Here's how the part is built. I have some questions about the finished solid (model axes, mm). A direction names the side the tool comes from. Give positions to 0.01 mm unless a question says otherwise; leave off trailing zeros. Loops run counter-clockwise (first coordinate to the right, second up) from the corner with the lowest first, then second, coordinate; pieces in that order, holes last.
Q1. I'm going to push flat-ended pins straight in: P1, Ø6.5, axis at y = -30, z = -30, coming from the +X side; P2, Ø11, axis at x = 51.5, z = -20.5, coming from the -Y side; P3, Ø4, axis at x = 51, y = -4.5, coming from the -Z side. Where does each tip first touch, or does it pass through?
Q2. For faces 1 (the face through (6, 35, 28.734)), 2 (the face through (16, 17.462, -24)), 3 (the face through (41.275, -8, 13)), which set-ups out of +Z, -Z, +X, -X, +Y, -Y let a thin tool reach every point of the face, with its end or its side?
Q3. I need wall thicknesses on probe 1 along Z at (x, y) = (37.5, -4.5) (1 decimal); probe 2 along Y at (x, z) = (19.5, -31.75); probe 3 along Z at (x, y) = (5.5, 26.5). Which ranges of each line are inside material? Lowest first, please.
Q4. Suppose I cut it at B-B (y = 2). List the corners of the cut face in (x, z) for me (1 decimal), and give its area (3 significant figures).
Q5. Suppose I cut it at A-A (z = 31.75). List the corners of the cut face in (x, y) for me (1 decimal), and give its area (3 significant figures).
Q6. Suppose I cut it at C-C (x = 52). Count the separate pieces of the cut face and the enclosed holes in it, and give its area (3 significant figures).
Q7. Thinking about a two-plate mould opening in Z: for faces 4 (the face through (41.275, -8, -12)), 5 (the face through (48.162, 22.907, 3.495)), 6 (the face through (36, 20.002, -25)), 7 (the face through (6, 28, 20.479)), which applies, pulls with the +Z half, pulls with the -Z half, needs draft (parallel to the pull), parting line crosses it, or undercut?
Autodesk Inventor part; units mm, degrees
ref_plane "YZ Plane" through (0, 0, 0) normal (1, 0, 0) x (0, 1, 0)
ref_plane "XZ Plane" through (0, 0, 0) normal (0, 1, 0) x (-1, 0, 0)
ref_plane "XY Plane" through (0, 0, 0) normal (0, 0, 1) x (1, 0, 0)
sketch "Sketch1" plane through (0, 0, 0) normal (1, 0, 0) x (0, 1, 0)
  line L0 (38.1, 38.1) -> (-38.1, 38.1)
  line L1 (-38.1, 38.1) -> (-38.1, -38.1)
  line L2 (-38.1, -38.1) -> (38.1, -38.1)
  line L3 (38.1, -38.1) -> (38.1, 38.1)
  point P0 (0, 0)
  dimension "d0" = 76.2
  dimension "d1" = 76.2
  dimension "d2" = 38.1
  dimension "d3" = 38.1
extrude "Extrusion1" add sketch "Sketch1" along normal blind 41.275
sketch "Sketch2" plane through (41.275, 0, 0) normal (1, 0, 0) x (0, 0, -1)
  line L0 (-38.1, -38.1) -> (38.1, -38.1)
  line L1 (38.1, -38.1) -> (38.1, 38.1)
  line L2 (38.1, 38.1) -> (-38.1, 38.1)
  line L3 (-38.1, 38.1) -> (-38.1, -38.1)
  line L4 (-34.925, 17.4625) -> (-14.2875, 17.4625)
  line L5 (-14.2875, 17.4625) -> (-14.2875, -26.9875)
  line L6 (-14.2875, -26.9875) -> (-34.925, -26.9875)
  line L7 (-34.925, -26.9875) -> (-34.925, 17.4625)
  dimension "d64" = 20.6375
  dimension "d65" = 44.45
  dimension "d66" = 3.175
  dimension "d67" = 11.1125
extrude "Extrusion2" cut sketch "Sketch2" against normal blind 39.6875 contours L4 L5 L6 L7
sketch "Sketch3" plane through (41.275, 0, 0) normal (1, 0, 0) x (0, 0, -1)
  line L0 (-14.2875, 17.4625) -> (-14.2875, -26.9875)
  line L1 (-14.2875, -26.9875) -> (-34.925, -26.9875)
  line L2 (-34.925, -26.9875) -> (-34.925, 17.4625)
  line L3 (-34.925, 17.4625) -> (-14.2875, 17.4625)
  line L4 (-38.1, -38.1) -> (38.1, -38.1)
  line L5 (38.1, -38.1) -> (38.1, 38.1)
  line L6 (38.1, 38.1) -> (-38.1, 38.1)
  line L7 (-38.1, 38.1) -> (-38.1, -38.1)
  line L8 (-14.2875, -26.9875) -> (-34.925, -26.9875)
  line L9 (-34.925, -26.9875) -> (-14.2875, -26.9875)
  line L10 (-14.2875, -26.9875) -> (-14.2875, -34.925)
  line L11 (-14.2875, -34.925) -> (-34.925, -34.925)
  line L12 (-34.925, -34.925) -> (-34.925, -26.9875)
  line L13 (-34.925, 17.4625) -> (-14.2875, 17.4625)
  line L14 (-14.2875, 17.4625) -> (-14.2875, 20.0025)
  line L15 (-14.2875, 20.0025) -> (-34.925, 20.0025)
  line L16 (-34.925, 20.0025) -> (-34.925, 17.4625)
  dimension "d68" = 7.9375
  dimension "d69" = 20.6375
  dimension "d70" = 20.6375
  dimension "d71" = 20.6375
  dimension "d72" = 2.54
extrude "Extrusion3" cut sketch "Sketch3" against normal blind 11.1125 contours L3 L16 L15 L14 | L10 L11 L12 L1
sketch "Sketch4" plane through (15.875, 17.4625, 12.7) normal (0, -1, 0) x (1, 0, 0)
  line L0 (-15.875, -50.8) -> (-15.875, 25.4)
  line L1 (-15.875, 25.4) -> (25.4, 25.4)
  line L2 (25.4, -50.8) -> (25.4, 25.4)
  line L3 (-15.875, -50.8) -> (25.4, -50.8)
  line L4 (25.4, 22.225) -> (25.4, 1.5875)
  line L5 (25.4, 22.225) -> (14.2875, 22.225)
  line L6 (14.2875, 22.225) -> (14.2875, 1.5875)
  line L7 (25.4, 1.5875) -> (14.2875, 1.5875)
  line L8 (-15.875, 16.0338) -> (-3.175, 16.0338)
  line L9 (-3.175, 16.0338) -> (-3.175, 7.7788)
  line L10 (-3.175, 7.7788) -> (-15.875, 7.7788)
  line L11 (-15.875, 7.7788) -> (-15.875, 16.0338)
  point P0 (-3.175, 11.9063)
  dimension "d73" = 8.255
  dimension "d74" = 12.7
  dimension "d75" = 20.6375
  dimension "d76" = 10.3187
extrude "Extrusion4" cut sketch "Sketch4" against normal blind 38.1 contours L0 L8 L9 L10
mirror "Mirror1" about plane through (0, 0, 0) normal (0, 0, 1) of "Extrusion4", "Extrusion3", "Extrusion2"
sketch "Sketch5" plane through (41.275, 0, 0) normal (1, 0, 0) x (0, 0, -1)
  line L0 (-38.1, -38.1) -> (38.1, -38.1)
  line L1 (38.1, -38.1) -> (38.1, 38.1)
  line L2 (38.1, 38.1) -> (-38.1, 38.1)
  line L3 (-38.1, 38.1) -> (-38.1, -38.1)
  line L4 (-38.1, -38.1) -> (38.1, -38.1)
  line L5 (-2.54, -38.1) -> (2.54, -38.1)
  line L6 (2.54, -38.1) -> (2.54, 20.6375)
  line L7 (2.54, 23.8125) -> (-2.54, 23.8125)
  line L8 (-2.54, 20.6375) -> (-2.54, -38.1)
  line L9 (-38.1, 38.1) -> (-38.1, -38.1)
  line L10 (38.1, 38.1) -> (-38.1, 38.1)
  line L11 (-38.1, 38.1) -> (-38.1, 23.8125)
  line L12 (-38.1, 23.8125) -> (-5.715, 23.8125)
  line L13 (38.1, 23.8125) -> (38.1, 38.1)
  line L14 (5.715, 23.8125) -> (38.1, 23.8125)
  line L15 (2.54, 23.8125) -> (2.54, 23.8125)
  arc A0 (-2.54, 20.6375) -> (-5.715, 23.8125) centre (-5.715, 20.6375) ccw
  arc A1 (5.715, 23.8125) -> (2.54, 20.6375) centre (5.715, 20.6375) ccw
  line L16 (-14.2875, 20.0025) -> (-14.2875, -34.925)
  line L17 (-34.925, -34.925) -> (-34.925, 20.0025)
  line L18 (-14.2875, -34.925) -> (-34.925, -34.925)
  line L19 (-34.925, 20.0025) -> (-14.2875, 20.0025)
  point P0 (0, 0)
  point P1 (38.1, 23.8125)
  point P2 (-2.54, -38.1)
  dimension "d36" = 5.08
  dimension "d39" = 2.54
  dimension "d40" = 3.175
  dimension "d44" = 61.9125
extrude "Extrusion5" add sketch "Sketch5" along normal blind 13.97 contours L8 A0 L12 L3 L2 L1 L14 A1 L6 L0
sketch "Sketch6" plane through (0, -38.1, 38.1) normal (0, 0, 1) x (1, 0, 0)
  line L0 (-11.1125, 84.1375) -> (53.975, 84.1375)
  line L1 (53.975, 84.1375) -> (53.975, -9.525)
  line L2 (53.975, -9.525) -> (-11.1125, -9.525)
  line L3 (-11.1125, -9.525) -> (-11.1125, 84.1375)
  point P0 (0, 38.1)
extrude "Extrusion6" [suppressed]
sketch "Sketch7" plane through (3.175, 22.225, -11.2395) normal (0, 0, -1) x (-1, 0, 0)
  line L0 (3.175, 15.875) -> (3.175, -60.325)
  line L1 (-28.575, 0) -> (-12.7, 0)
  line L2 (3.175, 15.875) -> (3.175, -60.325)
  line L3 (3.175, -60.325) -> (-38.1, -60.325)
  line L4 (-38.1, 1.5875) -> (-38.1, -60.325)
  line L5 (-38.1, 1.5875) -> (-52.07, 1.5875)
  line L6 (-52.07, 15.875) -> (-52.07, 1.5875)
  line L7 (3.175, 15.875) -> (-52.07, 15.875)
  line L8 (3.175, 15.875) -> (-6.35, 15.875)
  line L9 (-6.35, 15.875) -> (-6.35, 0)
  line L10 (-6.35, 0) -> (3.175, 0)
  line L11 (3.175, 0) -> (3.175, 15.875)
  line L12 (-6.35, -1.5875) -> (-6.35, 15.875)
  line L13 (-6.35, 0) -> (3.175, 12.7)
  point P0 (3.175, -22.225)
  point P1 (3.175, 15.875)
  point P2 (-6.35, 15.875)
  dimension "d49" = 9.525
  dimension "d50" = 3.175
extrude "Extrusion7" [suppressed]
mirror "Mirror2" [suppressed]
sketch "Sketch8" plane through (0, 38.1, 38.1) normal (0, 1, 0) x (1, 0, 0)
  line L0 (9.525, 46.1645) -> (0, 46.1645)
  line L1 (0, 36.6395) -> (9.525, 36.6395)
  line L2 (15.875, 47.625) -> (15.875, 60.579)
  arc A0 (0, 36.6395) -> (0, 46.1645) centre (-0.8069, 41.402) ccw
  line L3 (0, 46.1645) -> (0, 36.6395)
  point P0 (0, 38.1)
  point P1 (3.175, 49.3395)
  point P2 (3.175, 58.8645)
  dimension "d53" = 4.8304
extrude "Extrusion8" [suppressed]
mirror "Mirror3" [suppressed]
sketch "Sketch11" plane through (55.245, 0, 0) normal (1, 0, 0) x (0, 0, -1)
  circle A0 centre (-31.75, 30.9563) radius 3.429
  circle A1 centre (31.75, 30.9563) radius 3.429
  line L0 (5.715, 23.8125) -> (38.1, 23.8125)
  line L1 (38.1, 23.8125) -> (38.1, 38.1)
  line L2 (38.1, 38.1) -> (-38.1, 38.1)
  line L3 (-38.1, 38.1) -> (-38.1, 23.8125)
  line L4 (-38.1, 23.8125) -> (-5.715, 23.8125)
  arc A2 (-2.54, 20.6375) -> (-5.715, 23.8125) centre (-5.715, 20.6375) ccw
  line L5 (-2.54, 20.6375) -> (-2.54, -38.1)
  line L6 (-2.54, -38.1) -> (2.54, -38.1)
  line L7 (2.54, -38.1) -> (2.54, 20.6375)
  arc A3 (5.715, 23.8125) -> (2.54, 20.6375) centre (5.715, 20.6375) ccw
  point P0 (0, 0)
  point P1 (0, 38.1)
  dimension "d77" = 63.5
  dimension "d78" = 76.2
  dimension "d79" = 31.75
  dimension "d80" = 14.2875
  dimension "d81" = 7.1437
  dimension "d82" = 7.1437
  dimension "d83" = 6.858
  dimension "d84" = 6.858
extrude "Extrusion10" cut sketch "Sketch11" against normal through all contours A0 | A1
equation "\"d70\" = d69"
equation "\"d71\" = d69"
equation "\"d44\" = d43"
equation "\"d81\" = 0.5 * d80"
equation "\"d82\" = d81"
properties part number "Part_2_servobox"
Solutions:
1. P1: stops at x = 30.16
1. P2: stops at y = 23.81
1. P3: stops at z = -2.54
2. face 1: -X, +Y
2. face 2: +X
2. face 3: +Z, +X, -Y
3. probe 1: z = -38.1 to -34.9, -14.3 to 14.3, 34.9 to 38.1
3. probe 2: y = -38.1 to -26.99, 17.46 to 27.53, 34.39 to 38.1
3. probe 3: z = -38.1 to -28.73, -20.48 to 20.48, 28.73 to 38.1
4. outline: (0, -38.1) - (41.3, -38.1) - (41.3, -34.9) - (1.6, -34.9) - (1.6, -14.3) - (41.3, -14.3) - (41.3, -2.5) - (55.2, -2.5) - (55.2, 2.5) - (41.3, 2.5) - (41.3, 14.3) - (1.6, 14.3) - (1.6, 34.9) - (41.3, 34.9) - (41.3, 38.1) - (0, 38.1) - close
4. area: 1,580 mm2
5. outline: (0, -38.1) - (41.3, -38.1) - (41.3, -34.9) - (30.2, -34.9) - (30.2, -27) - (1.6, -27) - (1.6, 17.5) - (30.2, 17.5) - (30.2, 20) - (41.3, 20) - (41.3, 23.8) - (55.2, 23.8) - (55.2, 27.5) - (0, 27.5) - close; (0, 34.4) - (55.2, 34.4) - (55.2, 38.1) - (0, 38.1) - close
5. area: 1,090 mm2
6. separate pieces: 1
6. enclosed holes: 2
6. area: 1,330 mm2
7. face 4: needs draft
7. face 5: pulls with the +Z half
7. face 6: undercut
7. face 7: undercut
